Geometry: final body of the model. Coordinates: model frame, mm. Face numbers are marked on the shaded views. A direction names the side the tool comes from. Coordinates: 2 decimals unless noted, no trailing zeros. Write each loop counter-clockwise with the first axis right and the second up, starting at its lowest first coordinate (ties: lowest second). Pieces come first, ordered by that corner, then holes. Notation, with made-up numbers: (2, 24) - (6, 24) arc R26 ccw to (6, 41) - close; hole circle Ø4 at (-34.75, 26.5). An arc over 180 degrees is marked (long way). Put each result on its own line as item: value.
```python
from build123d import *

# Parameters (mm, degrees)
SKETCH1_W           = 42
SKETCH1_H           = 25
BOSS_EXTRUDE1_DEPTH = 2
BOSS_EXTRUDE2_DEPTH = 2
SKETCH2_R           = 4
CUT_EXTRUDE1_DEPTH  = 2
SKETCH3_W           = 8
SKETCH3_H           = 2
BOSS_EXTRUDE3_DEPTH = 23


with BuildPart() as part:
    # Sketch1 → Boss-Extrude1 (new body)
    with BuildSketch(Plane(origin=(0, 0, 0), x_dir=(1, 0, 0), z_dir=(0, 1, 0))):
        with Locations((-21, 12.5)):
            Rectangle(SKETCH1_W, SKETCH1_H)
    extrude(amount=BOSS_EXTRUDE1_DEPTH)

    # 3DSketch1 → Boss-Extrude2 (add)
    with BuildSketch(Plane(origin=(0, 2, -25), x_dir=(-0.8575119035010357, 0.5144641244577025, 0), z_dir=(0, 0, -1))):
        Polygon((0, 0), (3.086784747, 5.145071421), (-3.773310481, 9.260784417), (8.573828506, 29.841070101), (15.433923734, 25.725357105), (12.861603111, 21.437797588), (15.434138822, 19.894405214), (19.035387693, 25.896988539), (49.905816556, 7.376279856), (46.304567685, 1.373696531), (48.877103396, -0.169695842), (51.449424018, 4.117863675), (58.308228487, 0), (45.962379922, -20.578134802), (39.102284694, -16.462421806), (36.015499947, -21.607493227), align=None)
    extrude(amount=-BOSS_EXTRUDE2_DEPTH)

    # Sketch2 → Cut-Extrude1 (cut)
    with BuildSketch(Plane.XY.offset(-23)):
        with Locations((-11, 22)):
            Circle(SKETCH2_R)
    extrude(amount=-CUT_EXTRUDE1_DEPTH, mode=Mode.SUBTRACT)

    # Sketch3 → Boss-Extrude3 (add)
    with BuildSketch(Plane.XY.offset(-23)):
        Polygon((-50, 31.997491717), (-50, 29.997491717), (-42.000000393, 29.997491717), (-42.000000393, 32), align=None)
        with Locations((4, 31)):
            Rectangle(SKETCH3_W, SKETCH3_H)
    extrude(amount=BOSS_EXTRUDE3_DEPTH)


solid = part.part
```
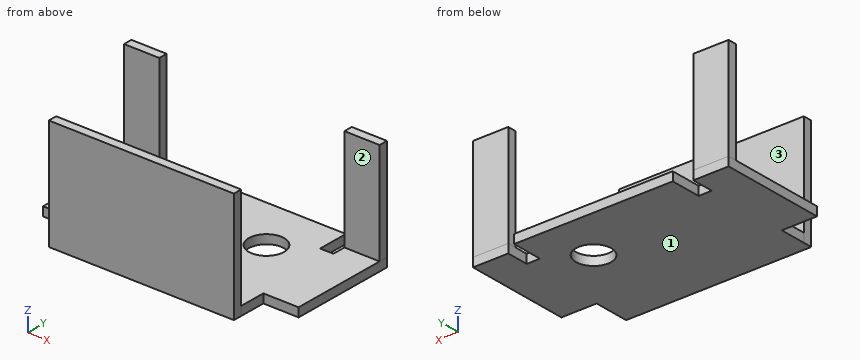
1. Pin query (flat end, axial travel): pin 1 Ø6.5 at (x, z) = (4, -14.5) entering from +Y; pin 2 Ø3 at (x, z) = (-16.5, -6) entering from +Y; pin 3 Ø12 at (x, z) = (-29.5, -9.5) entering from -Y; pin 4 Ø10 at (x, y) = (-26, 26) entering from +Z. Return the tip coordinate at first contact, or that it passes through.
Answer below:
pin 1: stops at y = 32
pin 2: stops at y = 2
pin 3: stops at y = 0
pin 4: stops at z = -23
2. Section query B-B (z = -20). Return loops of the section in (x, y), then the cut area to 3 significant figures.
Answer below:
outline: (-50, 30) - (-42, 30) - (-42, 32) - (-50, 32) - close; (-42, 0) - (0, 0) - (0, 2) - (-42, 2) - close; (0, 30) - (8, 30) - (8, 32) - (0, 32) - close
area: 116 mm²
3. Section query D-D (y = 28.5). Return loops of the section in (x, z).
Answer below:
outline: (-50, -25) - (-42, -25) - (-42, -23) - (-50, -23) - close; (-39, -25) - (-3, -25) - (-3, -23) - (-39, -23) - close; (0, -25) - (8, -25) - (8, -23) - (0, -23) - close
4. Section query A-A (y = 22). Return loops of the section in (x, z).
Answer below:
outline: (-50, -25) - (-15, -25) - (-15, -23) - (-50, -23) - close; (-7, -25) - (8, -25) - (8, -23) - (-7, -23) - close
5. Section query C-C (x = -11). Return loops of the section in (y, z).
Answer below:
outline: (0, -25) - (18, -25) - (18, -23) - (2, -23) - (2, 0) - (0, 0) - close; (26, -25) - (34, -25) - (34, -23) - (26, -23) - close
6. Set-up query: the marked faces 1, 2 and 3. Return all of +Z, -Z, +X, -X, +Y, -Y with unobstructed straight access to the full face (end or side cutting, diameter ignored); none if empty.
Answer below:
face 1: -Z, +X, -X, +Y, -Y
face 2: +Z, +X, -X, -Y
face 3: +Z, +X, -X, +Y
7. Ray query, probe 1 along Y at (x, z) = (-11, -24.55); probe 2 along Z at (x, y) = (-7, 7); probe 3 along Y at (x, z) = (-18, -20.25). Return the intervals inside material, ascending. Write a range as from..to.
Answer below:
probe 1: y = 0..18, 26..34
probe 2: z = -25..-23
probe 3: y = 0..2
